```python
from build123d import *

# Parameters (mm, degrees)
SKETCH2_R              = 3.5
SKETCH2_R_2            = 2.0955
BOSS_EXTRUDE1_DEPTH    = 5
BOSS_EXTRUDE1_2_DEPTH  = 5
SKETCH2_R_3            = 2.1
BOSS_EXTRUDE1_3_DEPTH  = 5
BOSS_EXTRUDE1_4_DEPTH  = 5
BOSS_EXTRUDE1_5_DEPTH  = 5
BOSS_EXTRUDE1_6_DEPTH  = 5
BOSS_EXTRUDE1_7_DEPTH  = 5
BOSS_EXTRUDE1_8_DEPTH  = 5
BOSS_EXTRUDE1_9_DEPTH  = 5
BOSS_EXTRUDE1_10_DEPTH = 5
BOSS_EXTRUDE2_DEPTH    = 3.175
BOSS_EXTRUDE3_DEPTH    = 25.4
BOSS_EXTRUDE4_DEPTH    = 16
BOSS_EXTRUDE5_DEPTH    = 3.175
BOSS_EXTRUDE6_DEPTH    = 31.75
SKETCH4_5_W            = 3.175
SKETCH4_5_H            = 105.156
BOSS_EXTRUDE7_DEPTH    = 4
BOSS_EXTRUDE8_DEPTH    = 3.175


with BuildPart() as part:
    # Sketch2 → Boss-Extrude1 (new body)
    with BuildSketch(Plane(origin=(0, 0, 32.776775543), x_dir=(-1, 0, 0), z_dir=(0, 0, -1))):
        with Locations((46.17832863, 161.386626861)):
            Circle(SKETCH2_R)
        with Locations((46.17832863, 161.386626861)):
            Circle(SKETCH2_R_2, mode=Mode.SUBTRACT)
    extrude(amount=BOSS_EXTRUDE1_DEPTH)



with BuildPart() as body_2:
    # Sketch2 → Boss-Extrude1 2 (new body)
    with BuildSketch(Plane(origin=(0, 0, 32.776775543), x_dir=(-1, 0, 0), z_dir=(0, 0, -1))):
        with Locations((96.17832863, 161.386626861)):
            Circle(SKETCH2_R)
        with Locations((96.17832863, 161.386626861)):
            Circle(SKETCH2_R_2, mode=Mode.SUBTRACT)
    extrude(amount=BOSS_EXTRUDE1_2_DEPTH)


with BuildPart() as body_3:
    # Sketch2 → Boss-Extrude1 3 (new body)
    with BuildSketch(Plane(origin=(0, 0, 32.776775543), x_dir=(-1, 0, 0), z_dir=(0, 0, -1))):
        with Locations((105.49632863, 162.322626861)):
            Circle(SKETCH2_R)
        with Locations((105.49632863, 162.322626861)):
            Circle(SKETCH2_R_3, mode=Mode.SUBTRACT)
    extrude(amount=BOSS_EXTRUDE1_3_DEPTH)


with BuildPart() as body_4:
    # Sketch2 → Boss-Extrude1 4 (new body)
    with BuildSketch(Plane(origin=(0, 0, 32.776775543), x_dir=(-1, 0, 0), z_dir=(0, 0, -1))):
        with Locations((218.52632863, 162.322626861)):
            Circle(SKETCH2_R)
        with Locations((218.52632863, 162.322626861)):
            Circle(SKETCH2_R_3, mode=Mode.SUBTRACT)
    extrude(amount=BOSS_EXTRUDE1_4_DEPTH)


with BuildPart() as body_5:
    # Sketch2 → Boss-Extrude1 5 (new body)
    with BuildSketch(Plane(origin=(0, 0, 32.776775543), x_dir=(-1, 0, 0), z_dir=(0, 0, -1))):
        with Locations((46.17832863, 88.136626861)):
            Circle(SKETCH2_R)
        with Locations((46.17832863, 88.136626861)):
            Circle(SKETCH2_R_2, mode=Mode.SUBTRACT)
    extrude(amount=BOSS_EXTRUDE1_5_DEPTH)


with BuildPart() as body_6:
    # Sketch2 → Boss-Extrude1 6 (new body)
    with BuildSketch(Plane(origin=(0, 0, 32.776775543), x_dir=(-1, 0, 0), z_dir=(0, 0, -1))):
        with Locations((46.17832863, 31.386626861)):
            Circle(SKETCH2_R)
        with Locations((46.17832863, 31.386626861)):
            Circle(SKETCH2_R_2, mode=Mode.SUBTRACT)
    extrude(amount=BOSS_EXTRUDE1_6_DEPTH)


with BuildPart() as body_7:
    # Sketch2 → Boss-Extrude1 7 (new body)
    with BuildSketch(Plane(origin=(0, 0, 32.776775543), x_dir=(-1, 0, 0), z_dir=(0, 0, -1))):
        with Locations((96.17832863, 31.386626861)):
            Circle(SKETCH2_R)
        with Locations((96.17832863, 31.386626861)):
            Circle(SKETCH2_R_2, mode=Mode.SUBTRACT)
    extrude(amount=BOSS_EXTRUDE1_7_DEPTH)


with BuildPart() as body_8:
    # Sketch2 → Boss-Extrude1 8 (new body)
    with BuildSketch(Plane(origin=(0, 0, 32.776775543), x_dir=(-1, 0, 0), z_dir=(0, 0, -1))):
        with Locations((96.17832863, 88.136626861)):
            Circle(SKETCH2_R)
        with Locations((96.17832863, 88.136626861)):
            Circle(SKETCH2_R_2, mode=Mode.SUBTRACT)
    extrude(amount=BOSS_EXTRUDE1_8_DEPTH)


with BuildPart() as body_9:
    # Sketch2 → Boss-Extrude1 9 (new body)
    with BuildSketch(Plane(origin=(0, 0, 32.776775543), x_dir=(-1, 0, 0), z_dir=(0, 0, -1))):
        with Locations((105.49632863, 69.358626861)):
            Circle(SKETCH2_R)
        with Locations((105.49632863, 69.358626861)):
            Circle(SKETCH2_R_3, mode=Mode.SUBTRACT)
    extrude(amount=BOSS_EXTRUDE1_9_DEPTH)


with BuildPart() as body_10:
    # Sketch2 → Boss-Extrude1 10 (new body)
    with BuildSketch(Plane(origin=(0, 0, 32.776775543), x_dir=(-1, 0, 0), z_dir=(0, 0, -1))):
        with Locations((218.52632863, 69.358626861)):
            Circle(SKETCH2_R)
        with Locations((218.52632863, 69.358626861)):
            Circle(SKETCH2_R_3, mode=Mode.SUBTRACT)
    extrude(amount=BOSS_EXTRUDE1_10_DEPTH)


with BuildPart() as part_1:
    add(part.part)

    add(body_2.part)  # Boss-Extrude2 merges body 2

    add(body_3.part)  # Boss-Extrude2 merges body 3

    add(body_4.part)  # Boss-Extrude2 merges body 4

    add(body_5.part)  # Boss-Extrude2 merges body 5

    add(body_6.part)  # Boss-Extrude2 merges body 6

    add(body_7.part)  # Boss-Extrude2 merges body 7

    add(body_8.part)  # Boss-Extrude2 merges body 8

    add(body_9.part)  # Boss-Extrude2 merges body 9

    add(body_10.part)  # Boss-Extrude2 merges body 10
    # Sketch3 → Boss-Extrude2 (add)
    with BuildSketch(Plane(origin=(0, 0, 27.776775543), x_dir=(-1, 0, 0), z_dir=(0, 0, -1))):
        Polygon((41.17832863, 166.386626861), (229.95632863, 166.386626861), (229.95632863, 61.230626861), (101.17832863, 61.230626861), (101.17832863, 26.386626861), (41.17832863, 26.386626861), (41.17832863, 61.230626861), align=None)
    extrude(amount=BOSS_EXTRUDE2_DEPTH)

    # Sketch4 → Boss-Extrude3 (add)
    with BuildSketch(Plane(origin=(0, 0, 24.601775543), x_dir=(-1, 0, 0), z_dir=(0, 0, -1))):
        Polygon((233.13132863, 61.230626861), (229.95632863, 61.230626861), (144.520113107, 61.230626861), (144.520113107, 58.055626861), (233.13132863, 58.055626861), align=None)
    extrude(amount=-BOSS_EXTRUDE3_DEPTH)

    # Sketch4<3> → Boss-Extrude4 (add)
    with BuildSketch(Plane(origin=(0, 0, 24.601775543), x_dir=(-1, 0, 0), z_dir=(0, 0, -1))):
        Polygon((144.520113107, 61.230626861), (144.520113107, 58.055626861), (233.13132863, 58.055626861), (233.13132863, 61.230626861), (229.95632863, 61.230626861), align=None)
    extrude(amount=-BOSS_EXTRUDE4_DEPTH)

    # Sketch5 → Boss-Extrude5 (add)
    with BuildSketch(Plane(origin=(0, 0, 24.601775543), x_dir=(-1, 0, 0), z_dir=(0, 0, -1))):
        Polygon((166.051482846, 58.055626861), (166.051482846, 48.055626861), (178.051482846, 48.055626861), (178.051482846, 51.055626861), (170.051482846, 51.055626861), (170.051482846, 55.055626861), (178.051482846, 55.055626861), (178.051482846, 58.055626861), align=None)
    extrude(amount=-BOSS_EXTRUDE5_DEPTH)

    # Sketch4<4> → Boss-Extrude6 (add)
    with BuildSketch(Plane(origin=(0, 0, 24.601775543), x_dir=(-1, 0, 0), z_dir=(0, 0, -1))):
        Polygon((41.17832863, 169.561626861), (41.17832863, 166.386626861), (229.95632863, 166.386626861), (233.13132863, 166.386626861), (233.13132863, 169.561626861), align=None)
    extrude(amount=-BOSS_EXTRUDE6_DEPTH)

    # Sketch4<5> → Boss-Extrude7 (add)
    with BuildSketch(Plane(origin=(0, 0, 24.601775543), x_dir=(-1, 0, 0), z_dir=(0, 0, -1))):
        with Locations((231.54382863, 113.808626861)):
            Rectangle(SKETCH4_5_W, SKETCH4_5_H)
    extrude(amount=-BOSS_EXTRUDE7_DEPTH)

    # Sketch6 → Boss-Extrude8 (add)
    with BuildSketch(Plane(origin=(0, 0, 24.601775543), x_dir=(-1, 0, 0), z_dir=(0, 0, -1))):
        Polygon((71.17832863, 169.561626861), (83.17832863, 169.561626861), (83.17832863, 172.561626861), (75.17832863, 172.561626861), (75.17832863, 176.561626861), (83.17832863, 176.561626861), (83.17832863, 179.561626861), (71.17832863, 179.561626861), align=None)
        Polygon((157.15482863, 179.561626861), (157.15482863, 169.561626861), (169.15482863, 169.561626861), (169.15482863, 172.561626861), (161.15482863, 172.561626861), (161.15482863, 176.561626861), (169.15482863, 176.561626861), (169.15482863, 179.561626861), align=None)
    extrude(amount=-BOSS_EXTRUDE8_DEPTH)


solid = part_1.part
```
CAD build for the part. Positions are in the model's coordinates, mm. A direction names the side the tool comes from. Give positions to 0.01 mm unless a question says otherwise; leave off trailing zeros. Order: outer loops, then holes, each group sorted by start corner. A loop starts at its lowest first (then second) coordinate and runs counter-clockwise, first axis right, second up.
(1) Saw through at D-D, the plane y = 130. Give the cut face in (x, z), then the cut area to 3 significant figures.
(2) Saw through at A-A, the plane z = 36. Give the cut face in (x, y).
(3) Drill centre lines: L1, parallel to Y at x = -146, z = 30; L2, parallel to X at y = 53, z = 27; L3, parallel to Z at x = -174.5, y = 155. Where is each one in solid material? Low to high.
(4) Saw through at B-B, the plane x = -175. Give the cut face in (y, z).
(5) Saw through at C-C, the plane x = -153.5. Give the cut face in (y, z), then the cut area to 3 significant figures.
(6) Tool access for faces 1 (the flat face through (-221, 69, 32.777)), 2 (the flat face through (-96.13, 85.85, 32.777)), 3 (the cylindrical face through (-45.72, 159.34, 30.31)): list every direction of +Z, -Z, +X, -X, +Y, -Y with a clear straight run to the whole face (end or side of a thin tool).
(7) Flat gauge pins, fed straight in: pin 1 (4.5 mm diameter, centred on x = -95.5, y = 161, fed in from +Z); pin 2 (3.5 mm diameter, centred on x = -173.5, z = 26, fed in from -Y); pin 3 (1.5 mm diameter, centred on x = -188.5, y = 129.5, fed in from +Z); pin 4 (12 mm diameter, centred on y = 90.5, z = 39.5, fed in from -X). Where does each tip first touch, or does it go through?
Results found:
1. outline: (-233.13, 24.6) - (-41.18, 24.6) - (-41.18, 27.78) - (-229.96, 27.78) - (-229.96, 28.6) - (-233.13, 28.6) - close
1. area: 612 mm2
2. outline: (-233.13, 58.06) - (-144.52, 58.06) - (-144.52, 61.23) - (-233.13, 61.23) - close; (-233.13, 166.39) - (-41.18, 166.39) - (-41.18, 169.56) - (-233.13, 169.56) - close
3. L1: y = 58.06 to 61.23, 166.39 to 169.56
3. L2: x = -170.05 to -166.05, -101.18 to -41.18
3. L3: z = 24.6 to 27.78
4. outline: (48.06, 24.6) - (51.06, 24.6) - (51.06, 27.78) - (48.06, 27.78) - close; (55.06, 24.6) - (169.56, 24.6) - (169.56, 56.35) - (166.39, 56.35) - (166.39, 27.78) - (61.23, 27.78) - (61.23, 50) - (58.06, 50) - (58.06, 27.78) - (55.06, 27.78) - close
5. outline: (58.06, 24.6) - (169.56, 24.6) - (169.56, 56.35) - (166.39, 56.35) - (166.39, 27.78) - (61.23, 27.78) - (61.23, 50) - (58.06, 50) - close
5. area: 515 mm2
6. face 1: +Z, +X, -X
6. face 2: +Z, +X, -X, -Y
6. face 3: +Z
7. pin 1: stops at z = 32.78
7. pin 2: stops at y = 48.06
7. pin 3: stops at z = 27.78
7. pin 4: passes through
